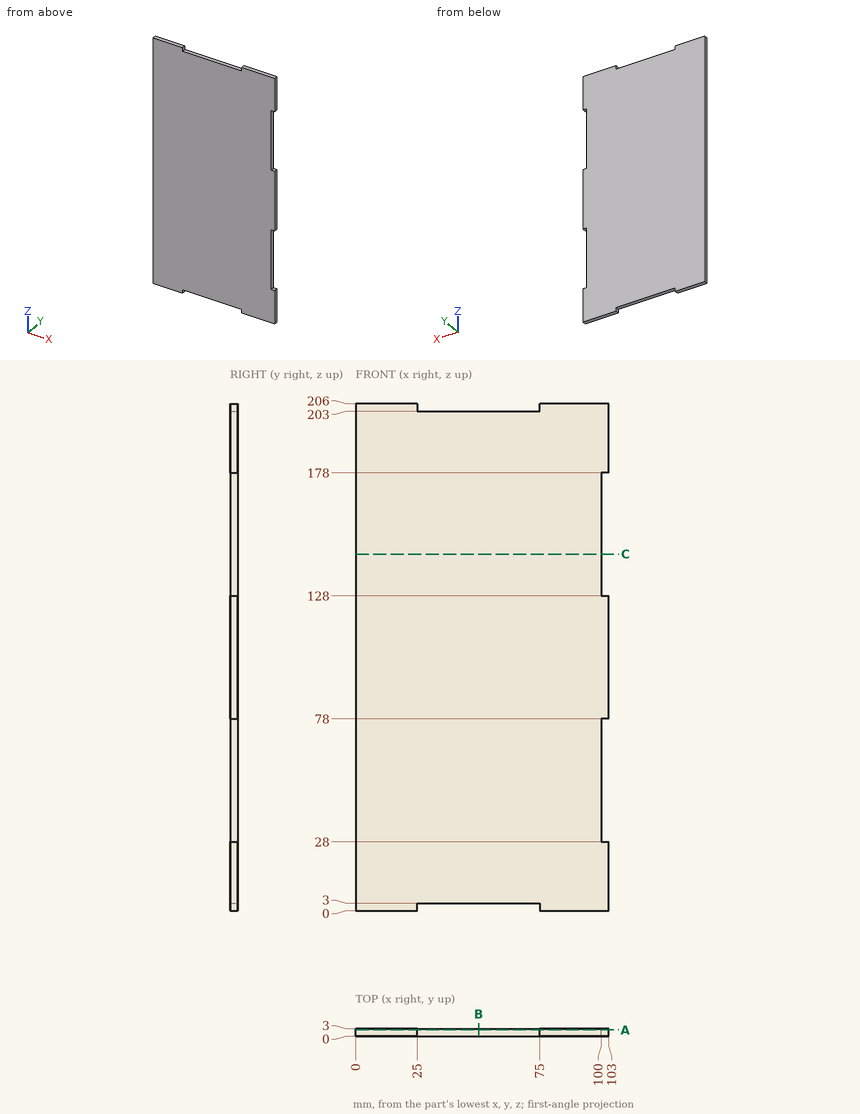
The figure shows three views and two pictorial views of one solid part (mm, origin at its lowest corner). Answer the questions. Round coordinates to 2 decimals unless told otherwise and drop trailing zeros. Write each loop counter-clockwise with the first axis right and the second up, starting at its lowest first coordinate (ties: lowest second). Pieces come first, ordered by that corner, then holes. Notation, with made-up numbers: M -2,47.25 L 21,47.25 A18 ccw 21,55.25 Z; hole C 12.25,78 d9. An arc over 180 degrees is marked long. Use a Markdown table: item, result.
1) The part is cut by section B-B (x = 50). Write down the section's boundary in (y, z), plus the area to 3 significant figures.
Answers follow:
| item | result |
|---|---|
| outline | M 0,3 L 3,3 L 3,203 L 0,203 Z |
| area | 600 mm2 |
2) The part is cut by section C-C (z = 145). Write down the section's boundary in (x, y), plus the area to 3 significant figures.
Answers follow:
| item | result |
|---|---|
| outline | M 0,0 L 100,0 L 100,3 L 0,3 Z |
| area | 300 mm2 |
3) Flat-ended cylindrical pins translate along their axes: pin 1 (2 mm diameter, centred on x = 72.5, z = 123, fed in from -Y); pin 2 (1.5 mm diameter, centred on x = 38, y = 1, fed in from +Z); pin 3 (0.9 mm diameter, centred on y = 1.5, z = 153, fed in from +X); pin 4 (0.9 mm diameter, centred on x = 51.5, y = 2, fed in from -Z). Find the tip coordinate at first contact, or state that the pin passes through.
Answers follow:
| item | result |
|---|---|
| pin 1 | stops at y = 0 |
| pin 2 | stops at z = 203 |
| pin 3 | stops at x = 100 |
| pin 4 | stops at z = 3 |
4) Straight lines are drawn through the part: line 1 along Z through (x, y) = (49, 2.3); line 2 along X through (y, z) = (2.4, 77.5). For each, find the intervals that lie inside material, in ascending order. Write a range as [from, to].
Answers follow:
| item | result |
|---|---|
| line 1 | z = [3, 203] |
| line 2 | x = [0, 100] |
5) The part is cut by section A-A (y = 2.45). Write down the section's boundary in (x, z), plus the area to 3 significant figures.
Answers follow:
| item | result |
|---|---|
| outline | M 0,0 L 25,0 L 25,3 L 75,3 L 75,0 L 103,0 L 103,28 L 100,28 L 100,78 L 103,78 L 103,128 L 100,128 L 100,178 L 103,178 L 103,206 L 75,206 L 75,203 L 25,203 L 25,206 L 0,206 Z |
| area | 20,600 mm2 |
